For this review, take the finished solid that the model builds, in its own axes (mm). Face numbers are marked on the shaded views. A direction names the side the tool comes from. Round coordinates to 2 decimals unless told otherwise and drop trailing zeros. Loops run counter-clockwise (first coordinate to the right, second up) from the corner with the lowest first, then second, coordinate; pieces in that order, holes last. Notation, with made-up numbers: M 42.5,37.25 L 95.5,37.25 A13 cw 95.5,43.25 Z; hole C -13,7 d9. An arc over 180 degrees is marked long. One line per question, with ' | ' between items. Start each with the question number.
1) For probe 1 along Z at (x, y) = (14, -3); probe 2 along Y at (x, z) = (0, -7.25) (3 decimals); probe 3 along Y at (x, z) = (-7, -1.75), list the stretches that pass through material, from the lowest coordinate up. Write a range as from..to.
2) For pin 1 Ø8 at (x, y) = (6.5, -6.5) entering from -Z; pin 2 Ø1 at (y, z) = (9.5, -4) entering from -X; pin 3 Ø5 at (x, z) = (3.5, -4) entering from +Y; pin 4 Ø1.5 at (x, z) = (0, -3.5) entering from -Y, all flat-tipped, find the tip position at first contact; note any pin that passes through.
3) Mouldability with a two-part tool opening along Z and no side actions: class the marked faces 1, 2 and 3 as pulls with the +Z half, pulls with the -Z half, needs draft (parallel to the pull), parting line crosses it, or undercut.
4) For the marked faces 4, 5, 6 and 7, list the 3-axis set-ups (+Z, -Z, +X, -X, +Y, -Y) from which the entire face can be reached by the end or side of a thin tool; tool diameter is ignored.
5) We need section A-A (x = 0). Give the boundary of the cut face in (y, z) (3 decimals), and give its area (3 significant figures).
```python
from build123d import *

# Parameters (mm, degrees)
CUT_EXTRUDE1_START = 2.2987
CUT_EXTRUDE1_DEPTH = 10.922
CIRPATTERN1_COUNT  = 16
SKETCH8_R          = 9.525
CUT_EXTRUDE2_DEPTH = 27.618169923


with BuildPart() as part:
    # Sketch2 → Revolve1 (revolve)
    with BuildSketch(Plane(origin=(0, 0, 0), x_dir=(0, 0, -1), z_dir=(1, 0, 0)), mode=Mode.PRIVATE) as revolve1_sk:
        with BuildLine():
            Line((-3.9878, 3.175), (10.3124, 3.175))
            Line((10.3124, 3.175), (10.3124, 15.875))
            Line((10.3124, 15.875), (9.46785, 15.875))
            ThreePointArc((9.46785, 15.875), (8.846219323, 15.130824061), (8.6233, 14.187145354))
            Line((8.6233, 14.187145354), (8.6233, 12.499290707))
            Line((8.6233, 12.499290707), (-2.2987, 12.499290707))
            Line((-2.2987, 12.499290707), (-2.2987, 14.187145354))
            ThreePointArc((-2.2987, 14.187145354), (-2.521619323, 15.130824061), (-3.14325, 15.875))
            Line((-3.14325, 15.875), (-3.9878, 15.875))
            Line((-3.9878, 15.875), (-3.9878, 8.7376))
            Line((-3.9878, 8.7376), (-3.9878, 3.175))
        make_face()
    revolve(revolve1_sk.sketch.rotate(Axis((0, 0, 10.3124), (0, 0, -1)), 90), axis=Axis((0, 0, 10.3124), (0, 0, -1)))

    # Sketch3 → Cut-Extrude1 (cut)
    with BuildSketch(Plane.XY.offset(CUT_EXTRUDE1_START)):
        with BuildLine():
            Line((-0.690489274, 11.1633), (0.690489274, 11.1633))
            Line((0.690489274, 11.1633), (1.2827, 12.4333))
            ThreePointArc((1.2827, 12.4333), (0, 12.499290707), (-1.2827, 12.4333))
            Line((-1.2827, 12.4333), (-0.690489274, 11.1633))
        make_face()
    cut_extrude1 = extrude(amount=-CUT_EXTRUDE1_DEPTH, mode=Mode.SUBTRACT)

    # CirPattern1: Cut-Extrude1 ×16 about axis
    cirpattern1_axis = Axis((0, 0, 0), (0, 0, 1))
    for i in range(1, CIRPATTERN1_COUNT):
        add(cut_extrude1.rotate(cirpattern1_axis, i * 360 / CIRPATTERN1_COUNT), mode=Mode.SUBTRACT)

    # Sketch8 → Cut-Extrude2 (cut, through all)
    with BuildSketch(Plane.XY.offset(3.9878)):
        Circle(SKETCH8_R)
    extrude(amount=-CUT_EXTRUDE2_DEPTH, mode=Mode.SUBTRACT)


solid = part.part
```
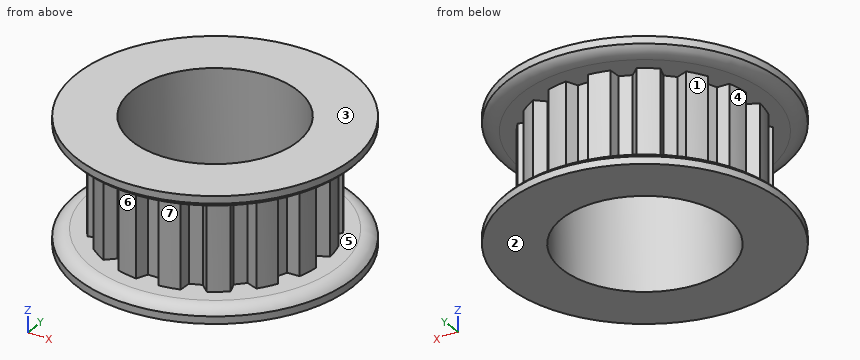
Answers below:
1) probe 1: -10.31..-8.63, 2.3..3.99 | probe 2: -11.163..-9.525, 9.525..11.163 | probe 3: -10.36..-6.46, 6.46..10.36
2) pin 1: z = -10.31 | pin 2: x = -7.88 | pin 3: y = 12.43 | pin 4: y = -11.29
3) face 1: undercut | face 2: pulls with the -Z half | face 3: pulls with the +Z half
4) face 4: -X, +Y | face 5: none | face 6: -X, -Y | face 7: +X, -Y
5) outline: M -15.875,-10.312 L -9.525,-10.312 L -9.525,3.988 L -15.875,3.988 L -15.875,3.143 A2.109 ccw -14.187,2.299 L -11.163,2.299 L -11.163,-8.623 L -14.187,-8.623 A2.109 ccw -15.875,-9.468 Z; M 9.525,-10.312 L 15.875,-10.312 L 15.875,-9.468 A2.109 ccw 14.187,-8.623 L 11.163,-8.623 L 11.163,2.299 L 14.187,2.299 A2.109 ccw 15.875,3.143 L 15.875,3.988 L 9.525,3.988 Z | area: 77.0 mm^2
